Source: CAD feature listing. Evaluate the final solid. Frame: model axes, mm. A direction names the side the tool comes from. Round coordinates to 2 decimals unless told otherwise and drop trailing zeros. Write each loop counter-clockwise with the first axis right and the second up, starting at its lowest first coordinate (ties: lowest second). Pieces come first, ordered by that corner, then holes. Notation, with made-up numbers: (84, -19) -> (109, -19) arc R13 cw to (109, 4) -> close; hole circle Ø11 at (22.5, -24). An arc over 180 degrees is marked (long way). Put each result on its own line as item: value.
Autodesk Inventor part; units mm, degrees
ref_plane "Work Plane1" through (0, 0, 150) normal (0, 0, -1) x (-1, 0, 0)
ref_plane "YZ Plane" through (0, 0, 0) normal (1, 0, 0) x (0, 1, 0)
ref_plane "XZ Plane" through (0, 0, 0) normal (0, 1, 0) x (-1, 0, 0)
sketch "Sketch1" plane through (0, 0, 0) normal (0, 0, 1) x (1, 0, 0)
  line L0 (-15, 15) -> (15, 15)
  line L1 (15, 15) -> (15, -15)
  line L2 (15, -15) -> (-15, -15)
  line L3 (-15, -15) -> (-15, 15)
  line L4 (12.5, 12.5) -> (-12.5, 12.5)
  line L5 (-12.5, 12.5) -> (-12.5, -12.5)
  line L6 (-12.5, -12.5) -> (12.5, -12.5)
  line L7 (12.5, -12.5) -> (12.5, 12.5)
  point P0 (0, 0)
  dimension "d0" = 30
  dimension "d1" = 30
  dimension "d2" = 15
  dimension "d3" = 15
  dimension "d4" = 2.5
extrude "Extrusion1" add sketch "Sketch1" along normal blind 1000
fillet "Fillet1" radius 2 4 edges at (15, 15, 500) (-15, 15, 500) (-15, -15, 500) (15, -15, 500)
ref_plane "Work Plane1" through (0, 0, 150) normal (0, 0, -1) x (-1, 0, 0)
split "Split1" [suppressed]
equation "\"d0\" = sm_varx_squareBarDimension"
equation "\"d1\" = d0"
equation "\"d4\" = sm_varx_squareBarThickness"
equation "\"sm_varx_squareBarDimension\" = 30"
equation "\"sm_varx_squareBarThickness\" = 2.5"
equation "\"hoop_angle_z\" = 45deg"
equation "\"hoop_bearing_length\" = 5deg"
equation "\"hoop_cable_diam\" = 5"
equation "\"hoop_cable_pulley_diam\" = 22"
equation "\"rack_tooth_addendum\" = 5"
equation "\"rack_tooth_dedendum\" = 5"
equation "\"rack_tooth_thickness\" = 5"
equation "\"secure_arm_angle\" = 20deg"
equation "\"secure_arm_hold_length\" = 35"
equation "\"secure_arm_radii\" = 9"
equation "\"support_baseClamp_platformLengthBuffer\" = 35"
equation "\"support_baseClamp_platformThickness\" = 15"
equation "\"support_baseClamp_platformWidthBuffer\" = 0"
equation "\"support_baseClamp_sleeveHoleDiameter\" = 12"
equation "\"support_baseClamp_sleeveSweepTerminationAngle\" = 55deg"
equation "\"support_baseClamp_thickness\" = 8"
equation "\"support_frame_endHoleBuffer\" = 25"
equation "\"support_frame_squareBarFillet\" = 2"
equation "\"support_frame_squareBarThickness\" = 5"
equation "\"hoop_tabs_thickness\" = 6"
equation "\"hoop_tabs_hole\" = 4"
equation "\"wheelchair_deployed_width\" = 635"
equation "\"wheelchair_deployed_length\" = 1067"
equation "\"wheelchair_deployed_height\" = 914"
properties part number "bar_steel_square_hollow_30x30x1000_2.5" material "Steel, Galvanized"
Q1. Draft query along X for faces 1 (the flat face through (-15, 0, 493)), 2 (the flat face through (0, 15, 493)), 3 (the flat face through (15, 0, 493)), 4 (the flat face through (12.5, 0, 493)). Return one class per face: +X half, -X half, draft (parallel to the pull), parting line (faces both ways), or undercut.
Ans:
face 1: -X half
face 2: draft
face 3: +X half
face 4: undercut
Q2. Reachability of faces 5 (the flat face through (-14, 0, 1000)), 6 (the flat face through (-12.5, 0, 493)) from +Z, -Z, +X, -X, +Y, -Y: full face, straight path, thin tool, end or side. Return the list, or none.
Ans:
face 5: +Z, +X, -X, +Y, -Y
face 6: +Z, -Z
Q3. Cut plane A-A on x = 7.5. Output: boundary loops of the cut face in (y, z), and give its area (3 significant figures).
Ans:
outline: (-15, 0) -> (-12.5, 0) -> (-12.5, 1000) -> (-15, 1000) -> close; (12.5, 0) -> (15, 0) -> (15, 1000) -> (12.5, 1000) -> close
area: 5,000 mm^2
Q4. Material intervals for line 1 (Y direction, x = -3.75, z = 284); line 2 (X direction, y = 13.5, z = 674.5), sorted ascending. Write a range as [from, to].
Ans:
line 1: y = [-15, -12.5], [12.5, 15]
line 2: x = [-14.94, 14.94]
Q5. Cut plane B-B on z = 454. Output: boundary loops of the cut face in (x, y), and give its area (3 significant figures).
Ans:
outline: (-15, -13) arc R2 ccw to (-13, -15) -> (13, -15) arc R2 ccw to (15, -13) -> (15, 13) arc R2 ccw to (13, 15) -> (-13, 15) arc R2 ccw to (-15, 13) -> close; hole (-12.5, -12.5) -> (12.5, -12.5) -> (12.5, 12.5) -> (-12.5, 12.5) -> close
area: 272 mm^2
Q6. Pin query (flat end, axial travel): pin 1 (12 mm diameter, centred on x = 1, y = -4.5, fed in from +Z). Return the tip coordinate at first contact, or that it passes through.
Ans:
pin 1: passes through
